Design review of the part built by this model. Coordinates are the model's own, in mm. Face numbers are marked on the shaded views. A direction names the side the tool comes from. Give positions to 0.01 mm unless a question says otherwise; leave off trailing zeros. Loops run counter-clockwise (first coordinate to the right, second up) from the corner with the lowest first, then second, coordinate; pieces in that order, holes last. Notation, with made-up numbers: (11, 7) -> (53, 7) arc R18 ccw to (53, 21) -> close; hole circle Ø1 at (27.25, 0.25). An arc over 180 degrees is marked (long way). Answer as CSV lines item,"result".
from build123d import *

# Parameters (mm, degrees)
F0_R          = 11
F1_DEPTH      = 44.45
F0_R_2        = 15.5
F2_DEPTH      = 3.175
F3_R          = 6.35
F4_DEPTH      = 9.525
F7_DEPTH      = 25.4
F7_DEPTH_BACK = 25.4
F8_R          = 3.175
F9_DEPTH      = 25.4
F10_SIZE      = 0.508


# Not quite as in the source:
# - a fillet or chamfer that OpenCascade refuses, or shapes differently, is made with other operations: its cross-section is extruded or revolved along the edge and cut away or added


with BuildPart() as f1:
    # F0 (on Front) → F1 (new body)
    with BuildSketch(Plane.XZ):
        Circle(F0_R)
    extrude(amount=F1_DEPTH)

    # F0 (on Front) → F2 (join)
    with BuildSketch(Plane.XZ):
        Circle(F0_R_2)
        Circle(F0_R, mode=Mode.SUBTRACT)
    extrude(amount=F2_DEPTH)

    # F3 (on face) → F4 (join)
    with BuildSketch(Plane.XZ.offset(44.45)):
        Circle(F3_R)
    extrude(amount=F4_DEPTH)

    # F5: fillet of radius 5.08 on 1 edges, made by hand

    # F5_s1 → F5_t2 (revolve, cut)
    with BuildSketch(Plane.XY):
        with BuildLine():
            ThreePointArc((11, -39.3882315343), (9.6610426354, -42.8249450807), (6.35, -44.45))
            Line((6.35, -44.45), (11, -44.45))
            Line((11, -44.45), (11, -39.3882315343))
        make_face()
    revolve(axis=Axis((0, -44.45, 0), (0, -1, 0)), mode=Mode.SUBTRACT)

    # F6 (on Top) → F7 (cut, two sides)
    with BuildSketch(Plane.XY) as f7_sk:
        with BuildLine():
            Line((-6.3399745388, -32.1066831191), (-6.3399745388, -31.3933168809))
            ThreePointArc((-6.3399745388, -31.3933168809), (-6.35, -31.75), (-6.3399745388, -32.1066831191))
        make_face()
        with BuildLine():
            Line((-6.3399745388, -18.1366831191), (-6.3399745388, -31.3933168809))
            Line((-6.3399745388, -31.3933168809), (-6.3399745388, -32.1066831191))
            ThreePointArc((-6.3399745388, -32.1066831191), (0, -38.1), (6.3399745388, -32.1066831191))
            Line((6.3399745388, -32.1066831191), (6.3399745388, -31.3933168809))
            Line((6.3399745388, -31.3933168809), (6.3399745388, -18.1366831191))
            Line((6.3399745388, -18.1366831191), (6.3399745388, -17.4233168809))
            ThreePointArc((6.3399745388, -17.4233168809), (0, -11.43), (-6.3399745388, -17.4233168809))
            Line((-6.3399745388, -17.4233168809), (-6.3399745388, -18.1366831191))
        make_face()
        with BuildLine():
            ThreePointArc((-6.3399745388, -17.4233168809), (-6.35, -17.78), (-6.3399745388, -18.1366831191))
            Line((-6.3399745388, -18.1366831191), (-6.3399745388, -17.4233168809))
        make_face()
        with BuildLine():
            Line((6.3399745388, -31.3933168809), (6.3399745388, -32.1066831191))
            ThreePointArc((6.3399745388, -32.1066831191), (6.35, -31.75), (6.3399745388, -31.3933168809))
        make_face()
        with BuildLine():
            ThreePointArc((6.3399745388, -18.1366831191), (6.35, -17.78), (6.3399745388, -17.4233168809))
            Line((6.3399745388, -17.4233168809), (6.3399745388, -18.1366831191))
        make_face()
    extrude(amount=-F7_DEPTH, mode=Mode.SUBTRACT)
    extrude(f7_sk.sketch, amount=F7_DEPTH_BACK, mode=Mode.SUBTRACT)

    # F8 (on face) → F9 (cut)
    with BuildSketch(Plane.XZ.offset(53.975)):
        Circle(F8_R)
    extrude(amount=-F9_DEPTH, mode=Mode.SUBTRACT)

    # F10
    f10_edges = [f1.edges().sort_by_distance(p)[0] for p in [
        (-15.5, -3.175, 0),
        (-6.35, -53.975, 0),
    ]]
    chamfer(f10_edges, length=F10_SIZE)


solid = f1.part
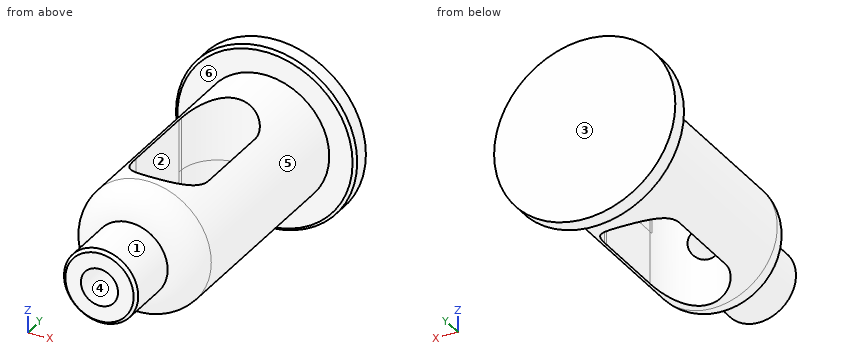
Q1. We need section C-C, the plane y = -49. State the section outline as (x, z) points (3 decimals).
Filled sheet:
outline,"circle Ø12.7 at (0, 0); hole circle Ø6.35 at (0, 0)"
Q2. For the marked faces 1, 2 and 3, list the 3-axis set-ups (+Z, -Z, +X, -X, +Y, -Y) from which the entire face can be reached by the end or side of a thin tool; tool diameter is ignored.
Filled sheet:
face 1,"-Y"
face 2,"+Z, -Z"
face 3,"+Z, -Z, +X, -X, +Y"
Q3. We need section A-A, the plane x = 0. State the section outline as (y, z) points (3 decimals).
Filled sheet:
outline,"(-53.975, -5.842) -> (-53.467, -6.35) -> (-44.45, -6.35) arc R5.08 ccw to (-39.388, -11) -> (-38.1, -11) -> (-38.1, -3.175) -> (-53.975, -3.175) -> close; (-53.975, 3.175) -> (-38.1, 3.175) -> (-38.1, 11) -> (-39.388, 11) arc R5.08 ccw to (-44.45, 6.35) -> (-53.467, 6.35) -> (-53.975, 5.842) -> close; (-11.43, -11) -> (-3.175, -11) -> (-3.175, -14.992) -> (-2.667, -15.5) -> (0, -15.5) -> (0, 15.5) -> (-2.667, 15.5) -> (-3.175, 14.992) -> (-3.175, 11) -> (-11.43, 11) -> close"
Q4. We need section D-D, the plane y = -7.5. State the section outline as (x, z) points.
Filled sheet:
outline,"circle Ø22 at (0, 0)"
Q5. To check wall thickness, follow probe 1 along Z at (x, y) = (0, -49) (3 decimals); probe 2 along Y at (x, z) = (-3.5, -4) (3 decimals); probe 3 along Y at (x, z) = (-1, 12) (3 decimals). State the ranges of each line that lie inside material, in increasing order. Write a range as from..to.
Filled sheet:
probe 1,"z = -6.35..-3.175, 3.175..6.35"
probe 2,"y = -53.975..-37.048, -12.482..0"
probe 3,"y = -3.175..0"
Q6. We need section B-B, the plane y = -25. State the section outline as (x, z) points, and give its area (3 significant figures).
Filled sheet:
outline,"(-6.34, -8.99) -> (-6.34, 8.99) arc R11 ccw to start; (6.34, -8.99) arc R11 ccw to (6.34, 8.99) -> close"
area,"117 mm^2"
Q7. Clearance check with flat-ended pins moving along their axes: pin 1 Ø10 at (y, z) = (-24.5, -2.5) entering from -X; pin 2 Ø2 at (y, z) = (-6, -7) entering from -X; pin 3 Ø3 at (y, z) = (-34.5, 3.5) entering from +X. State where each tip first meets the part, or that it passes through.
Filled sheet:
pin 1,"stops at x = -11"
pin 2,"stops at x = -9.22"
pin 3,"stops at x = 10.82"
Q8. The part is to be moulded in two halves that separate along X. For the marked faces 4, 5 and 6, say which applies: pulls with the +X half, pulls with the -X half, needs draft (parallel to the pull), parting line crosses it, or undercut.
Filled sheet:
face 4,"undercut"
face 5,"parting line crosses it"
face 6,"needs draft"
